Geometry check sheet. Reference: the model listing, model coordinates, mm. A direction names the side the tool comes from. Give positions to 0.01 mm unless a question says otherwise; leave off trailing zeros. Write each loop counter-clockwise with the first axis right and the second up, starting at its lowest first coordinate (ties: lowest second). Pieces come first, ordered by that corner, then holes. Notation, with made-up numbers: M -19,89 L 16,89 A27 ccw 16,111 Z; hole C 63,-28.75 d5. An arc over 180 degrees is marked long. Use one line per item in the form item = value. Start each with the question number.
```python
from build123d import *

# Parameters (mm, degrees)
F0_R        = 13
F1_DEPTH    = 6
F2_R        = 5
F3_DEPTH    = 21
F4_S5_R     = 5
F4_T6_DEPTH = 20
F5_R        = 13
F6_DEPTH    = 1
F8_R        = 1.6
F9_DEPTH    = 25
F10_R       = 2.55
F11_DEPTH   = 15
F12_R       = 2.05
F13_DEPTH   = 30


# Not quite as in the source:
# - a fillet or chamfer that OpenCascade refuses, or shapes differently, is made with other operations: its cross-section is extruded or revolved along the edge and cut away or added


with BuildPart() as f1:
    # F0 (on Top) → F1 (new body)
    with BuildSketch(Plane.XY):
        Circle(F0_R)
    extrude(amount=F1_DEPTH)

    # F2 (on face) → F3 (join)
    with BuildSketch(Plane.XY.offset(6)):
        Circle(F2_R)
    extrude(amount=F3_DEPTH)

    # F4: chamfer of 8 on 1 edges, made by hand


with BuildPart() as f4_tool2:
    # F4_s3 → F4_t4 (revolve)
    with BuildSketch(Plane.XZ):
        Polygon((13, -2), (5, 6), (13, 6), align=None)
    revolve(axis=Axis((0, 0, 6), (0, 0, 1)))

    # F4_s5 → F4_t6 (cut, symmetric)
    with BuildSketch(Plane.XY.offset(2)):
        Circle(F4_S5_R)
    extrude(amount=F4_T6_DEPTH, both=True, mode=Mode.SUBTRACT)


with BuildPart() as f1_1:
    add(f1.part)

    # F4_t1: cut F4_tool2
    add(f4_tool2.part, mode=Mode.SUBTRACT)

    # F5
    f5_edges = [f1_1.edges().sort_by_distance(p)[0] for p in [
        (-5, 0, 6),
    ]]
    fillet(f5_edges, radius=F5_R)

    # F6 (add): a face of the model
    f6_faces = [f1_1.faces().sort_by_distance(p)[0] for p in [
        (0, 0, 0),
    ]]
    extrude(f6_faces, amount=F6_DEPTH)

    # F8 (on offset) → F9 (cut)
    with BuildSketch(Plane(origin=(0, 0, 1.4), x_dir=(1, 0, 0), z_dir=(0, 0, -1))):
        with Locations((6.0621778265, -3.5)):
            Circle(F8_R)
        with Locations((0, 7)):
            Circle(F8_R)
        with Locations((-6.0621778265, -3.5)):
            Circle(F8_R)
    extrude(amount=F9_DEPTH, mode=Mode.SUBTRACT)

    # F10 (on offset) → F11 (cut)
    with BuildSketch(Plane(origin=(0, 0, 1.4), x_dir=(1, 0, 0), z_dir=(0, 0, -1))):
        with Locations((0, 7)):
            Circle(F10_R)
        with Locations((6.0621778265, -3.5)):
            Circle(F10_R)
        with Locations((-6.0621778265, -3.5)):
            Circle(F10_R)
    extrude(amount=-F11_DEPTH, mode=Mode.SUBTRACT)

    # F12 (on face) → F13 (cut)
    with BuildSketch(Plane.XY.offset(27)):
        Circle(F12_R)
    extrude(amount=-F13_DEPTH, mode=Mode.SUBTRACT)


solid = f1_1.part
```
(1) Sectioned sample at A-A, the plane x = 0. State how many separate pieces and enclosed holes the cut face has, plus the area to 3 significant figures.
(2) Tool access check on faces 1 (the cylindrical face through (4, 2, 7)), 2 (the cylindrical face through (4.77, 1.5, 19.08)), 3 (the flat face through (4.1, 2.4, 16.4)). Record the directions out of +Z, -Z, +X, -X, +Y, -Y that give a thin tool (end or side, any length) a straight path to the whole face; none if there is none.
(3) Thickness scan on probe 1 along Y at (x, z) = (0, -0.35); probe 2 along Y at (x, z) = (0, 12); probe 3 along X at (y, z) = (3.5, 0.25). Record the ranges inside material, lowest first. Write a range as [from, to].
(4) Depth check by flat-ended pin: pin 1 (8 mm diameter, centred on x = -6.5, z = 21, fed in from +Y); pin 2 (1 mm diameter, centred on x = 3, y = -7.5, fed in from +Z); pin 3 (1 mm diameter, centred on x = -5.5, y = 8, fed in from +Z). Enter the tip coordinate at first touch or a pass-through.
(5) Draft check along Z on faces 4 (the flat face through (-0.2, -2.3, -1)), 5 (the cylindrical face through (4.9, 2.4, 0.2)), 6 (the conical face through (8.234, -3.414, 2.086)), 7 (the flat face through (-4.1, 2.4, 16.4)). Enter one of: released by +Z, released by -Z, zero draft, split by the parting line, or undercut.
(6) Sectioned sample at B-B, the plane z = 15.75. Record the boundary of the cut face in (x, y), plus the area to 3 significant figures.
Numbers:
q1.separate_pieces = 3
q1.enclosed_holes = 0
q1.area = 190 mm2
q2.face_1 = none
q2.face_2 = +Z
q2.face_3 = +X, +Y
q3.probe_1 = [-11, -8.6], [-5.4, -2.05], [2.05, 11]
q3.probe_2 = [-4.45, -2.05], [2.05, 5]
q3.probe_3 = [-10.16, -7.66], [-4.46, 4.46], [7.66, 10.16]
q4.pin_1 = 4.33
q4.pin_2 = 3.61
q4.pin_3 = 1.79
q5.face_4 = released by -Z
q5.face_5 = zero draft
q5.face_6 = released by +Z
q5.face_7 = undercut
q6.outline = M -4.84,1.26 A5 ccw -1.32,-4.82 A2.55 cw 1.32,-4.82 A5 ccw 4.84,1.26 A2.55 cw 3.51,3.56 A5 ccw -3.51,3.56 A2.55 cw Z; hole C 0,0 d4.1
q6.area = 62.4 mm2
